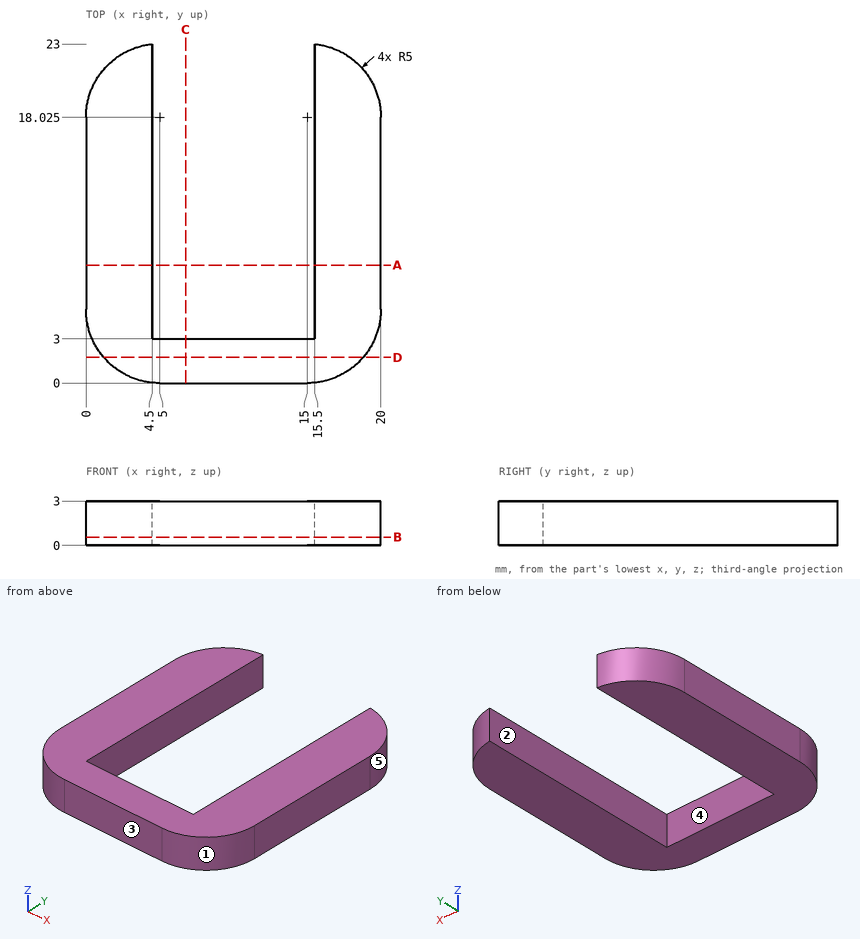
Study the drawing (mm; zero at the part's minimum x, y, z) and answer. A direction names the side the tool comes from. Give positions to 0.01 mm unless a question says otherwise; leave off trailing zeros. Loops run counter-clockwise (first coordinate to the right, second up) from the corner with the lowest first, then second, coordinate; pieces in that order, holes last. Notation, with made-up numbers: M -2.75,5 L 20.25,5 A31 ccw 20.25,41 Z; hole C 3.25,41.25 d6. An arc over 180 degrees is marked long. Answer as CSV lines item,"result".
Item 1: The part is cut by section D-D (y = 1.75). Give the vertices of the cut face in (x, z).
Values follow:
outline,"M 1.2,0 L 18.8,0 L 18.8,3 L 1.2,3 Z"
Item 2: Straight lines are drawn through the part: line 1 along X through (y, z) = (14, 0.65); line 2 along Y through (x, z) = (9.75, 0.9); line 3 along X through (y, z) = (22.25, 2.75). For each, find the intervals that lie inside material, in ascending order. Write a range as [from, to].
Values follow:
line 1,"x = [0, 4.5], [15.5, 20]"
line 2,"y = [0, 3]"
line 3,"x = [2.33, 4.5], [15.5, 17.67]"
Item 3: Given pin 1 Ø1.5 at (y, z) = (3.5, 1) entering from +X; pin 2 Ø12 at (x, y) = (13.5, 6.5) entering from +Z; pin 3 Ø0.9 at (x, z) = (8.5, 2) entering from +Y, each flat-ended and moving along its own axis, determine where each tip first touches the part or whether it passes through.
Values follow:
pin 1,"stops at x = 19.94"
pin 2,"stops at z = 3"
pin 3,"stops at y = 3"
Item 4: Which of the six approach directions +Z, -Z, +X, -X, +Y, -Y give full straight-line access (tool end or side, diameter ignored) to the marked faces 4 and 5?
Values follow:
face 4,"+Z, -Z, +Y"
face 5,"+Z, -Z, +X, +Y"
Item 5: The part is cut by section A-A (y = 8). Give the vertices of the cut face in (x, z), and give its area (3 significant figures).
Values follow:
outline,"M 0,0 L 4.5,0 L 4.5,3 L 0,3 Z; M 15.5,0 L 20,0 L 20,3 L 15.5,3 Z"
area,"27.0 mm^2"
Item 6: The mould has two halves that part along X. Classify the marked faces 1, 2 and 3: released by +X, released by -X, zero draft, split by the parting line, or undercut.
Values follow:
face 1,"released by +X"
face 2,"undercut"
face 3,"zero draft"
Item 7: The part is cut by section C-C (x = 6.75). Give the vertices of the cut face in (y, z), and give its area (3 significant figures).
Values follow:
outline,"M 0,0 L 3,0 L 3,3 L 0,3 Z"
area,"9.00 mm^2"
Item 8: The part is cut by section B-B (z = 0.55). Give the vertices of the cut face in (x, y) (3 decimals), and give its area (3 significant figures).
Values follow:
outline,"M 0,5 A5 ccw 5,0 L 15,0 A5 ccw 20,5 L 20,18.025 A5 ccw 15.5,23 L 15.5,3 L 4.5,3 L 4.5,23 A5 ccw 0,18.025 Z"
area,"219 mm^2"
